from build123d import *

# Parameters (mm, degrees)
EXTRUDE_1_DEPTH               = 0.5
FILLET_1_RADIUS               = 0.45
FILLET_1_LENGTH               = 0.5
CHAMFER_1_SIZE                = 0.5
FILLET_1_OF_MIRROR_1_2_RADIUS = 0.45
FILLET_1_OF_MIRROR_1_2_LENGTH = 0.5
CHAMFER_1_OF_MIRROR_1_SIZE    = 0.5
SKETCH_5_R                    = 1.25
EXTRUDE_2_DEPTH               = 53.5


with BuildPart() as part:
    # 草图1 → 凸台-拉伸1 (new body)
    with BuildSketch(Plane.XY):
        with BuildLine():
            Line((-2.344520595, -0.867884312), (-1, -4.5))
            Line((-1, -4.5), (-1, -14.5))
            Line((-1, -14.5), (0, -14.5))
            Line((0, -14.5), (0, -1.6))
            ThreePointArc((0, -1.6), (-1.13137085, -1.13137085), (-1.6, 0))
            Line((-1.6, 0), (-1.6, 4.6))
            Line((-1.6, 4.6), (-2.5, 4.6))
            Line((-2.5, 4.6), (-2.5, 0))
            ThreePointArc((-2.5, 0), (-2.460823184, -0.440850605), (-2.344520595, -0.867884312))
        make_face()
    extrude_1 = extrude(amount=EXTRUDE_1_DEPTH)

    # 圆角1: full round fillet: the end face becomes a half cylinder, R = half its width
    fillet_1_face = Plane((-2.05, 4.6, 0.25), x_dir=(0, 0, 1), z_dir=(0, 1, 0))  # on the end face: x along it, z out of the body
    fillet_1_slab = fillet_1_face.offset(-FILLET_1_RADIUS / 2) * Box(FILLET_1_LENGTH, 2 * FILLET_1_RADIUS, FILLET_1_RADIUS, mode=Mode.PRIVATE)  # the body's end, R deep
    fillet_1_round = Plane((-2.05, 4.15, 0.25), x_dir=(0, 1, 0), z_dir=(0, 0, 1)) * Cylinder(FILLET_1_RADIUS, FILLET_1_LENGTH, mode=Mode.PRIVATE)  # its axis R under the face
    add(fillet_1_slab - fillet_1_round, mode=Mode.SUBTRACT)

    # 倒角1
    chamfer_1_edges = [part.edges().sort_by_distance(p)[0] for p in [
        (-1, -9.5, 0.5),
    ]]
    chamfer(chamfer_1_edges, length=CHAMFER_1_SIZE - 0.0001)  # a hair under: the kernel refuses the full size

    # 镜向1: 凸台-拉伸1 across Right Plane
    add(extrude_1.mirror(Plane(origin=(0, 0, 0), x_dir=(0, 0, -1), z_dir=(1, 0, 0))))

    # 圆角1 of Mirror 1 2: full round fillet: the end face becomes a half cylinder, R = half its width
    fillet_1_of_mirror_1_2_face = Plane((2.05, 4.6, 0.25), x_dir=(0, 0, 1), z_dir=(0, 1, 0))  # on the end face: x along it, z out of the body
    fillet_1_of_mirror_1_2_slab = fillet_1_of_mirror_1_2_face.offset(-FILLET_1_OF_MIRROR_1_2_RADIUS / 2) * Box(FILLET_1_OF_MIRROR_1_2_LENGTH, 2 * FILLET_1_OF_MIRROR_1_2_RADIUS, FILLET_1_OF_MIRROR_1_2_RADIUS, mode=Mode.PRIVATE)  # the body's end, R deep
    fillet_1_of_mirror_1_2_round = Plane((2.05, 4.15, 0.25), x_dir=(0, 1, 0), z_dir=(0, 0, 1)) * Cylinder(FILLET_1_OF_MIRROR_1_2_RADIUS, FILLET_1_OF_MIRROR_1_2_LENGTH, mode=Mode.PRIVATE)  # its axis R under the face
    add(fillet_1_of_mirror_1_2_slab - fillet_1_of_mirror_1_2_round, mode=Mode.SUBTRACT)

    # 倒角1 of 镜向1
    chamfer_1_of_mirror_1_edges = [part.edges().sort_by_distance(p)[0] for p in [
        (1, -9.5, 0.5),
    ]]
    chamfer(chamfer_1_of_mirror_1_edges, length=CHAMFER_1_OF_MIRROR_1_SIZE - 0.0001)  # a hair under: the kernel refuses the full size

    # 草图3 → 旋转1 (revolve)
    with BuildSketch(Plane(origin=(0, 0, 0), x_dir=(0, 0, -1), z_dir=(1, 0, 0)), mode=Mode.PRIVATE) as revolve_1_sk:
        Polygon((2.5, -4.5), (2.5, -9.004043198), (3.1, -9.860932002), (3.1, -14.5), (2.6, -14.5), (2.6, -10.018581397), (2, -9.161692593), (2, -4.5), align=None)
    revolve(revolve_1_sk.sketch.rotate(Axis((0, -5.567856156, -0.6), (0, -1, 0)), 180), axis=Axis((0, -5.567856156, -0.6), (0, -1, 0)))

    # 草图5 → 凸台-拉伸2 (add)
    with BuildSketch(Plane(origin=(0, -4.5, 0), x_dir=(1, 0, 0), z_dir=(0, 1, 0))):
        with Locations(Location((0, 0.6, 0), (0, 0, 270))):
            Circle(SKETCH_5_R)
    extrude(amount=-EXTRUDE_2_DEPTH)


solid = part.part
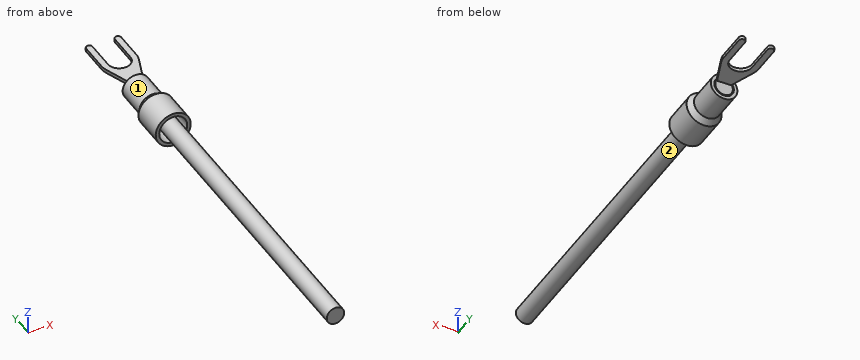
Model file for the job. Use its own axes, mm. Face numbers are marked on the shaded views. Give positions to 0.01 mm unless a question says otherwise; leave off trailing zeros. Order: outer loops, then holes, each group sorted by start corner. A loop starts at its lowest first (then second) coordinate and runs counter-clockwise, first axis right, second up. Notation, with made-up numbers: M 61.5,15 L 87.5,15 A14 ccw 87.5,39 Z; hole C -18.5,40.25 d7. An arc over 180 degrees is marked long. Put each result on its own line as item: value. Start each with the question number.
(1) Pin check, flat tips, straight feed: pin 1 Ø3 at (x, y) = (0, -44.5) entering from -Z; pin 2 Ø1 at (x, z) = (1.5, 1) entering from -Y; pin 3 Ø2 at (x, y) = (2, -51.5) entering from +Z. Stop position of each tip, or through.
(2) Band-saw the part on B-B on y = -41. Give the cut face in (x, z).
(3) Pull direction Z, two halves, no side cores. Call the marked faces 1 and 2: released by +Z, released by -Z, zero draft, split by the parting line, or undercut.
(4) Band-saw the part on A-A on z = -0.6. Give the cut face in (x, y).
(5) Drill centre lines: L1, parallel to X at y = -7.4, z = -0.6; L2, parallel to X at y = -11.95, z = -0.6; L3, parallel to X at y = 2.5, z = 0.05. Where is each one in solid material? Low to high. Write a range as [from, to].
Results below:
1. pin 1: stops at z = -1.85
1. pin 2: stops at y = -14.5
1. pin 3: stops at z = 0.15
2. outline: C 0,-0.6 d2.5
3. face 1: split by the parting line
3. face 2: undercut
4. outline: M -2.5,-14.5 L -2,-14.5 L -2,-10.02 L -1.4,-9.16 L -1.4,-4.5 L -1.9,-4.5 L -1.9,-9 L -2.5,-9.86 Z; M -1.25,-58 L 1.25,-58 L 1.25,-4.5 L -1.25,-4.5 Z; M 1.4,-9.16 L 2,-10.02 L 2,-14.5 L 2.5,-14.5 L 2.5,-9.86 L 1.9,-9 L 1.9,-4.5 L 1.4,-4.5 Z
5. L1: x = [-1.9, -1.4], [-1.25, 1.25], [1.4, 1.9]
5. L2: x = [-2.5, -2], [-1.25, 1.25], [2, 2.5]
5. L3: x = [-2.5, -1.6], [1.6, 2.5]
